```python
from build123d import *

# Parameters (mm, degrees)
SKETCH2_R          = 13.8938
SKETCH2_R_2        = 7.8994
SKETCH5_R          = 10.668
CUT_EXTRUDE1_DEPTH = 19.05
SKETCH6_R          = 10.668
CUT_EXTRUDE2_DEPTH = 19.05


with BuildPart() as part:
    # Sweep1: sweep along a path in Sketch3
    with BuildLine(Plane.XY) as sweep1_path:
        Line((-17.960512242, -17.960512242), (-4.490128061, -4.490128061))
        ThreePointArc((-4.490128061, -4.490128061), (-1.166946263, 0.483364969), (0, 6.35))
        Line((0, 6.35), (0, 25.4))
    # Sketch2 → Sweep1 (sweep)
    with BuildSketch(Plane(origin=(0, 25.4, 0), x_dir=(1, 0, 0), z_dir=(0, 1, 0))):
        Circle(SKETCH2_R)
        Circle(SKETCH2_R_2, mode=Mode.SUBTRACT)
    sweep(path=sweep1_path.line)

    # Sketch5 → Cut-Extrude1 (cut)
    with BuildSketch(Plane(origin=(0, 25.4, 0), x_dir=(1, 0, 0), z_dir=(0, 1, 0))):
        with Locations(Location((0, 0, 0), (0, 0, 270))):
            Circle(SKETCH5_R)
    extrude(amount=-CUT_EXTRUDE1_DEPTH, mode=Mode.SUBTRACT)

    # Sketch6 → Cut-Extrude2 (cut)
    with BuildSketch(Plane(origin=(-17.960512242, -17.960512242, 0), x_dir=(0, 0, 1), z_dir=(-0.7071067811865408, -0.7071067811865543, 0))):
        with Locations(Location((0, 0, 0), (0, 0, 270))):
            Circle(SKETCH6_R)
    extrude(amount=-CUT_EXTRUDE2_DEPTH, mode=Mode.SUBTRACT)


solid = part.part
```
The listing builds one solid part. Answer for the finished solid, in the listing's coordinates (mm). A direction names the side the tool comes from. Round coordinates to 2 decimals unless told otherwise and drop trailing zeros. Loops run counter-clockwise (first coordinate to the right, second up) from the corner with the lowest first, then second, coordinate; pieces in that order, holes last.
Q1. Section D-D, the plane z = -5.75 is taken. Determine the outline of the cut face in (x, y).
Q2. Find the intervals of material crossed by line 1 (X direction, y = 13.75, z = 0); line 2 (Y direction, x = -9.5, z = -5); line 3 (X direction, y = 4, z = -3.5), in increasing order.
Q3. Given pin 1 Ø10 at (y, z) = (-3, -9) entering from -X; pin 2 Ø1 at (y, z) = (5, -3.5) entering from +X; pin 3 Ø1 at (x, z) = (-15, 4) entering from -Y, each flat-ended and moving along its own axis, determine where each tip first touches the part or whether it passes through.
Q4. Section B-B, the plane y = 18 is taken. Determine the outline of the cut face in (x, z), then the cut area to 3 significant figures.
Q5. Section A-A, the plane z = 0 is taken. Determine the outline of the cut face in (x, y).
Q6. Section C-C, the plane z = -10 is taken. Determine the outline of the cut face in (x, y).
Q7. Which of the six approach directions +Z, -Z, +X, -X, +Y, -Y give full straight-line access (tool end or side, diameter ignored) to faces 1 (the face through (-9.55, 0.57, -3.9)), 2 (the face through (-6.491, 16.008, -8.466))?
Q8. For a pull along X with two mould halves and no side action, classify faces 3 (the face through (-4.351, -18.288, -4.086)), 4 (the face through (-15.095, -20.826, 10.227)), 5 (the face through (-10.2, 25.4, 4.1)) as released by +X, released by -X, zero draft, split by the parting line, or undercut.
Completed:
1. outline: (-26.9, -9.02) - (-24.31, -11.61) - (-10.84, 1.86) - (-8.32, -0.66) arc R9.91 ccw to (-5.42, 6.35) - (-8.99, 6.35) - (-8.99, 25.4) - (-12.65, 25.4) - (-12.65, 6.35) arc R2.68 cw to (-13.43, 4.45) - close; (-11.61, -24.31) - (-9.02, -26.9) - (4.45, -13.43) arc R27.98 ccw to (12.65, 6.35) - (12.65, 25.4) - (8.99, 25.4) - (8.99, 6.35) - (5.42, 6.35) arc R20.75 cw to (-0.66, -8.32) - (1.86, -10.84) - close
2. line 1: x = -13.89 to -10.67, 10.67 to 13.89
2. line 2: y = -26.42 to -22.83, 0.52 to 25.4
2. line 3: x = -15.02 to -7.42, 6.96 to 13.35
3. pin 1: stops at x = -24.73
3. pin 2: stops at x = 13.54
3. pin 3: stops at y = -1.6
4. outline: circle Ø27.79 at (0, 0); hole circle Ø21.34 at (0, 0)
4. area: 249 mm2
5. outline: (-27.78, -8.14) - (-25.5, -10.42) - (-12.03, 3.05) - (-10.08, 1.1) arc R7.43 ccw to (-7.9, 6.35) - (-10.67, 6.35) - (-10.67, 25.4) - (-13.89, 25.4) - (-13.89, 6.35) arc R1.44 cw to (-14.31, 5.33) - close; (-10.42, -25.5) - (-8.14, -27.78) - (5.33, -14.31) arc R29.22 ccw to (13.89, 6.35) - (13.89, 25.4) - (10.67, 25.4) - (10.67, 6.35) - (7.9, 6.35) arc R23.23 cw to (1.1, -10.08) - (3.05, -12.03) - close
6. outline: (-24.78, -11.14) - (-20.59, -15.33) - (-7.12, -1.86) - (-1.86, -7.12) - (-15.33, -20.59) - (-11.14, -24.78) - (2.33, -11.31) arc R24.98 ccw to (9.65, 6.35) - (9.65, 25.4) - (3.72, 25.4) - (3.72, 6.35) - (-3.72, 6.35) - (-3.72, 25.4) - (-9.65, 25.4) - (-9.65, 6.35) arc R5.68 cw to (-11.31, 2.33) - close
7. face 1: none
7. face 2: +Y
8. face 3: undercut
8. face 4: released by -X
8. face 5: zero draft
